Read the model definition and answer for the solid it produces. Units are mm, in the model's axes. Face numbers are marked on the shaded views. A direction names the side the tool comes from. Give positions to 0.01 mm unless a question says otherwise; leave off trailing zeros. Loops run counter-clockwise (first coordinate to the right, second up) from the corner with the lowest first, then second, coordinate; pieces in that order, holes last. Notation, with made-up numbers: (-33.75, 32) -> (-4.75, 32) arc R31 cw to (-4.75, 70) -> close; hole circle Ø4 at (22.25, 40). An arc over 180 degrees is marked (long way). Answer as CSV lines item,"result". Start each with the question number.
```python
from build123d import *

# Parameters (mm, degrees)
F1_ANGLE = 180
F3_DEPTH = 76.2


with BuildPart() as f1:
    # F0 (on Front) → F1 (revolve, symmetric)
    with BuildSketch(Plane.XZ) as f1_sk:
        with BuildLine():
            Line((-30.48, -3.81), (-30.48, 0))
            ThreePointArc((-30.48, 0), (-35.56, 3.962134), (-40.64, 0))
            Line((-40.64, 0), (-40.64, -3.81))
            Line((-40.64, -3.81), (-30.48, -3.81))
        make_face()
    revolve(axis=Axis((0, 0, 31.664096), (0, 0, 1)), revolution_arc=F1_ANGLE / 2)
    revolve(f1_sk.sketch, axis=Axis((0, 0, 31.664096), (0, 0, -1)), revolution_arc=F1_ANGLE / 2)

    # F2 (on Front) → F3 (cut, symmetric)
    with BuildSketch(Plane.XZ):
        Polygon((-5.08, -1.957448), (-8.953226, 14.028987), (-13.816583, 12.528193), (-10.306973, -1.957448), align=None)
    extrude(amount=F3_DEPTH, both=True, mode=Mode.SUBTRACT)


solid = f1.part
```
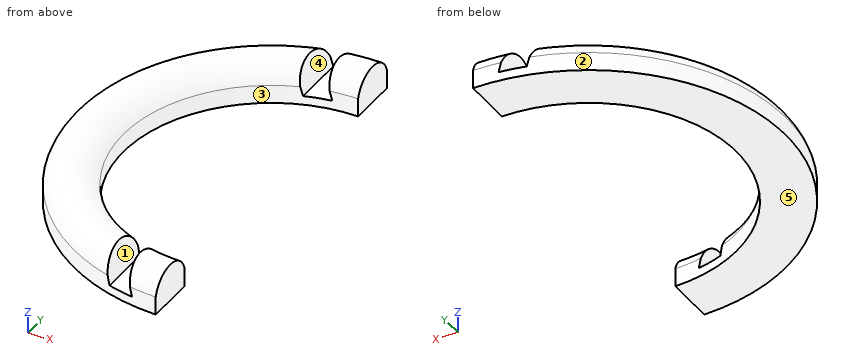
(1) Find section B-B on y = 0. Write down the section's boundary in (x, z).
(2) Find section A-A on z = 0.75. Write down the section's boundary in (x, y).
(3) Find the intervals of material crossed by line 1 along X through (y, z) = (-33, 0.25); line 2 along Y through (x, z) = (-16.5, -2); line 3 along Y through (x, z) = (-21, 1), in increasing order. Write a range as from..to.
(4) Each of these flat-tipped pins is pushed along its axis until it touches: P1, Ø2.5, axis at x = -7.5, y = -34, coming from the +Z side; P2, Ø1, axis at y = 2, z = 1.5, coming from the +X side; P3, Ø2, axis at y = 15, z = 0, coming from the -X side. Where does it stop, or does it pass through?
(5) A tool of negligible diameter and unlimited length cuts with its end or side. For the marked faces 1 and 2, from which of +Z, -Z, +X, -X, +Y, -Y can it reach the whole face along a straight path? Write none if from no direction.
(6) The mould has two halves that part along X. Classify the marked faces 3, 4 and 5: pulls with the +X half, pulls with the -X half, needs draft (parallel to the pull), parting line crosses it, or undercut.
Answer block:
1,outline,"(-40.64, -3.81) -> (-30.48, -3.81) -> (-30.48, 0) arc R5.24 ccw to (-40.64, 0) -> close"
2,outline,"(-10.96, -38.87) -> (-10.96, -28.71) arc R30.73 cw to (-10.96, 28.71) -> (-10.96, 38.87) arc R40.39 ccw to start; (-5.74, -39.98) arc R40.39 ccw to (0, -40.39) -> (0, -30.73) arc R30.73 cw to (-5.74, -30.19) -> close; (-5.74, 30.19) arc R30.73 cw to (0, 30.73) -> (0, 40.39) arc R40.39 ccw to (-5.74, 39.98) -> close"
3,line 1,"x = -23.6..-10.84, -5.61..0"
3,line 2,"y = -37.14..-25.63, 25.63..37.14"
3,line 3,"y = -34.37..-22.59, 22.59..34.37"
4,P1,"stops at z = 3.96"
4,P2,"stops at x = -30.78"
4,P3,"stops at x = -38.15"
5,face 1,"+Z, +Y, -Y"
5,face 2,"+Z, -Z, -X"
6,face 3,"pulls with the +X half"
6,face 4,"undercut"
6,face 5,"needs draft"
